from build123d import *

# Parameters (mm, degrees)
F0_W     = 50.8
F0_H     = 50.8
F1_DEPTH = 12.7
F2_R     = 7.124416
F3_DEPTH = 6.35
F2_R_2   = 7.81729
F4_DEPTH = 6.35
F2_R_3   = 7.053422
F5_DEPTH = 6.35
F2_R_4   = 9.132211
F6_DEPTH = 6.35


with BuildPart() as f1:
    # F0 (on Top) → F1 (new body)
    with BuildSketch(Plane.XY):
        Rectangle(F0_W, F0_H)
    extrude(amount=F1_DEPTH)

    # F2 (on face) → F3 (join)
    with BuildSketch(Plane.XY.offset(12.7)):
        with Locations((-13.650993, 12.323814)):
            Circle(F2_R)
    extrude(amount=F3_DEPTH)

    # F2 (on face) → F4 (join)
    with BuildSketch(Plane.XY.offset(12.7)):
        with Locations((12.134215, 12.703009)):
            Circle(F2_R_2)
    extrude(amount=F4_DEPTH)

    # F2 (on face) → F5 (join)
    with BuildSketch(Plane.XY.offset(12.7)):
        with Locations((-12.892607, -10.427844)):
            Circle(F2_R_3)
    extrude(amount=F5_DEPTH)

    # F2 (on face) → F6 (join)
    with BuildSketch(Plane.XY.offset(12.7)):
        with Locations((13.650997, -12.703009)):
            Circle(F2_R_4)
    extrude(amount=F6_DEPTH)


solid = f1.part
Geometry check sheet. Reference: the model listing, model coordinates, mm. A direction names the side the tool comes from. Coordinates: 2 decimals unless noted, no trailing zeros. Order: outer loops, then holes, each group sorted by start corner. A loop starts at its lowest first (then second) coordinate and runs counter-clockwise, first axis right, second up. Notation, with made-up numbers: (-9, 13.5) - (42, 13.5) arc R8 ccw to (42, 19.5) - close; hole circle Ø1 at (-33.5, -2.5). An arc over 180 degrees is marked (long way). Answer in a Markdown table with one row per item. Add a question column.
1) Cross-section at C-C, the plane y = -5. Record the cut outline in (x, z).
2) Set-up check for faces 1 (the cylindrical face through (10.44, 5.07, 15.83)), 2 (the flat face through (0, 25.4, 6)): record each of +Z, -Z, +X, -X, +Y, -Y from which the full face is reachable in a straight line by a thin tool's end or side.
3) Release check for a two-part mould opening along Y. For faces 3 (the cylindrical face through (-19.94, -10.12, 15.83)), 4 (the cylindrical face through (-6.856, 14.464, 15.831)), 5 (the flat face through (0, -25.4, 6)), 6 (the flat face through (-25.4, 0, 6)) record: +Y half, -Y half, draft (parallel to the pull), parting line (faces both ways), or undercut.
4) Cross-section at A-A, the plane x = 2.5. Record the cut outline in (y, z).
5) Material ranges on line 1 along Z through (x, y) = (0, 4.5); line 2 along Y through (x, z) = (5.5, 16.75); line 3 along Y through (x, z) = (13, 15), recorded low to high. Write a range as [from, to].
6) Gauge pin test, flat end, axial feed: P1, Ø4, axis at x = -10.5, y = 3, coming from the +Z side. Record the tip position at first contact, or that the pin passes through.
7) Cross-section at B-B, the plane z = 17.25. Record the cut outline in (x, y), then the cut area to 3 significant figures.
Check result:
| question | item | result |
|---|---|---|
| 1 | outline | (-25.4, 0) - (25.4, 0) - (25.4, 12.7) - (18.56, 12.7) - (18.56, 19.05) - (8.75, 19.05) - (8.75, 12.7) - (-8.39, 12.7) - (-8.39, 19.05) - (-17.4, 19.05) - (-17.4, 12.7) - (-25.4, 12.7) - close |
| 2 | face 1 | +Z |
| 2 | face 2 | +Z, -Z, +X, -X, +Y |
| 3 | face 3 | undercut |
| 3 | face 4 | undercut |
| 3 | face 5 | -Y half |
| 3 | face 6 | draft |
| 4 | outline | (-25.4, 0) - (25.4, 0) - (25.4, 12.7) - (-25.4, 12.7) - close |
| 5 | line 1 | z = [0, 12.7] |
| 5 | line 2 | y = [-16.82, -8.58], [8.57, 16.84] |
| 5 | line 3 | y = [-21.81, -3.59], [4.93, 20.47] |
| 6 | P1 | stops at z = 12.7 |
| 7 | outline | circle Ø14.25 at (-13.65, 12.32); circle Ø14.11 at (-12.89, -10.43); circle Ø15.63 at (12.13, 12.7); circle Ø18.26 at (13.65, -12.7) |
| 7 | area | 770 mm² |
